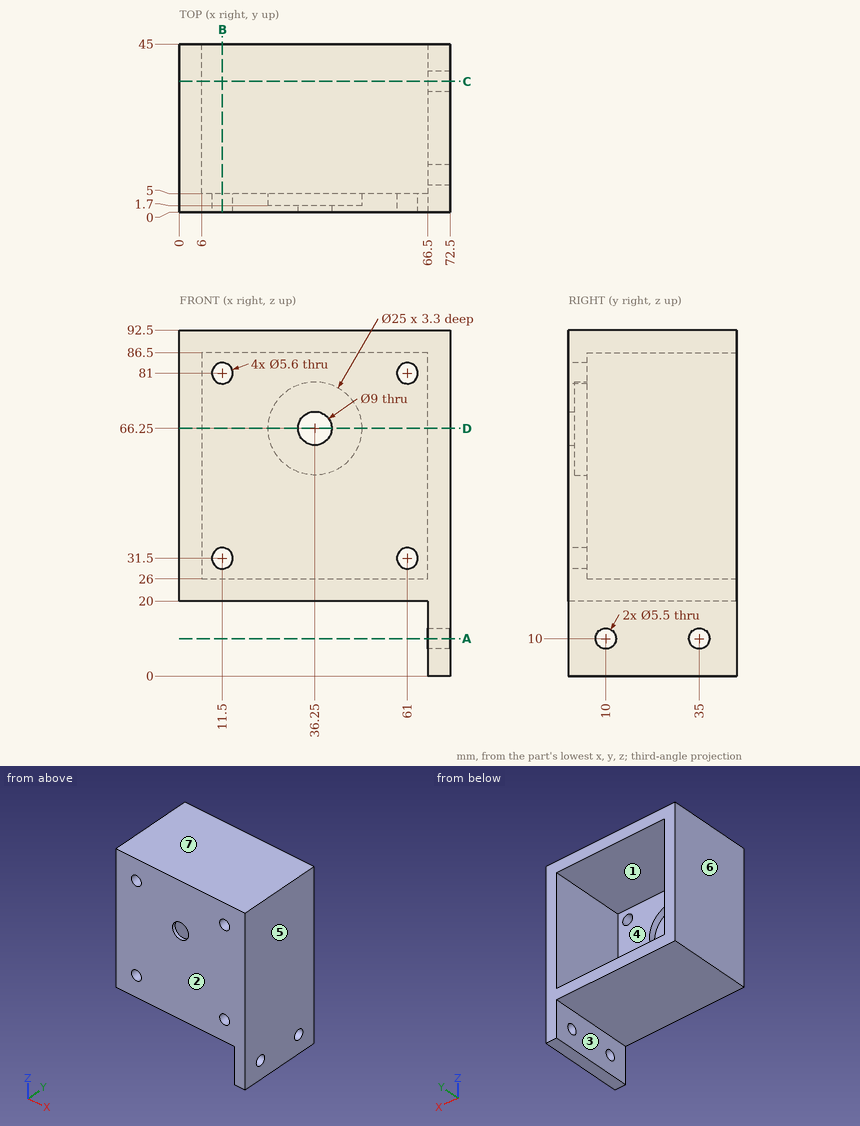
Study the drawing (mm; zero at the part's minimum x, y, z) and answer. A direction names the side the tool comes from. Round coordinates to 2 decimals unless told otherwise and drop trailing zeros. Write each loop counter-clockwise with the first axis right and the second up, starting at its lowest first coordinate (ties: lowest second). Pieces come first, ordered by that corner, then holes.
1) A cutting plane is placed at B-B on x = 11.5. Determine the outline of the cut face in (y, z), and give its area (4 significant figures).
2) Flat-ended cylindrical pins translate along their axes: P1, Ø20, axis at x = 32.5, y = 33, coming from the -Z side; P2, Ø6.5, axis at x = 11.5, z = 31.5, coming from the +Y side; P3, Ø7.5, axis at x = 30, z = 69, coming from the +Y side; P4, Ø1, axis at y = 27, z = 48, coming from the -X side. Find the tip coordinate at first contact, or state that the pin passes through.
3) A cutting plane is placed at A-A on z = 10. Determine the outline of the cut face in (x, y).
4) A cutting plane is placed at C-C on y = 35. Determine the outline of the cut face in (x, z).
5) Consider probe 1 along Z at (x, y) = (61, 2.4); probe 2 along Z at (x, y) = (62, 35.5); probe 3 along Y at (x, z) = (67, 10). Determine where each line is inside the solid, lowest interval first.
6) Determine the mould class of the marked faces 4, 5, 6 and 7 for opening direction X: pulls with the +X half, pulls with the -X half, needs draft (parallel to the pull), parting line crosses it, or undercut.
7) A cutting plane is placed at D-D on z = 66.25. Determine the outline of the cut face in (x, y).
8) Which of the six approach directions +Z, -Z, +X, -X, +Y, -Y give full straight-line access (tool end or side, diameter ignored) to the marked faces 1, 2 and 3?
Entries:
1. outline: (0, 20) - (45, 20) - (45, 26) - (5, 26) - (5, 28.7) - (0, 28.7) - close; (0, 34.3) - (5, 34.3) - (5, 78.2) - (0, 78.2) - close; (0, 83.8) - (5, 83.8) - (5, 86.5) - (45, 86.5) - (45, 92.5) - (0, 92.5) - close
1. area: 786.5 mm2
2. P1: stops at z = 20
2. P2: stops at y = 5
2. P3: stops at y = 1.7
2. P4: stops at x = 0
3. outline: (66.5, 0) - (72.5, 0) - (72.5, 7.25) - (66.5, 7.25) - close; (66.5, 12.75) - (72.5, 12.75) - (72.5, 32.25) - (66.5, 32.25) - close; (66.5, 37.75) - (72.5, 37.75) - (72.5, 45) - (66.5, 45) - close
4. outline: (0, 20) - (66.5, 20) - (66.5, 12.75) - (72.5, 12.75) - (72.5, 92.5) - (0, 92.5) - close; (66.5, 0) - (72.5, 0) - (72.5, 7.25) - (66.5, 7.25) - close; hole (6, 26) - (66.5, 26) - (66.5, 86.5) - (6, 86.5) - close
5. probe 1: z = 20 to 28.7, 34.3 to 78.2, 83.8 to 92.5
5. probe 2: z = 20 to 26, 86.5 to 92.5
5. probe 3: y = 0 to 7.25, 12.75 to 32.25, 37.75 to 45
6. face 4: undercut
6. face 5: pulls with the +X half
6. face 6: pulls with the -X half
6. face 7: needs draft
7. outline: (0, 0) - (31.75, 0) - (31.75, 1.7) - (23.75, 1.7) - (23.75, 5) - (6, 5) - (6, 45) - (0, 45) - close; (40.75, 0) - (72.5, 0) - (72.5, 45) - (66.5, 45) - (66.5, 5) - (48.75, 5) - (48.75, 1.7) - (40.75, 1.7) - close
8. face 1: +Y
8. face 2: +Z, -Z, +X, -X, -Y
8. face 3: -Z, -X, +Y, -Y
